```python
from build123d import *

# Parameters (mm, degrees)
SKETCH_1_R          = 3.15
EXTRUDE_1_DEPTH     = 2.15
SKETCH_2_R          = 2
EXTRUDE_2_DEPTH     = 35
CUT_EXTRUDE_1_DEPTH = 1.5


with BuildPart() as part:
    # 草图1 → 凸台-拉伸1 (new body)
    with BuildSketch(Plane(origin=(0, 0, 0), x_dir=(1, 0, 0), z_dir=(0, 1, 0))):
        Circle(SKETCH_1_R)
    extrude(amount=EXTRUDE_1_DEPTH)

    # 草图2 → 凸台-拉伸2 (add)
    with BuildSketch(Plane(origin=(0, 2.15, 0), x_dir=(1, 0, 0), z_dir=(0, 1, 0))):
        Circle(SKETCH_2_R)
    extrude(amount=EXTRUDE_2_DEPTH)

    # 草图3 → 切除-拉伸1 (cut)
    with BuildSketch(Plane.XZ):
        with BuildLine():
            Line((-0.5, 1), (-0.5, 2))
            Line((-0.5, 2), (0.5, 2))
            Line((0.5, 2), (0.5, 1))
            ThreePointArc((0.5, 1), (0.646446609, 0.646446609), (1, 0.5))
            Line((1, 0.5), (2, 0.5))
            Line((2, 0.5), (2, -0.5))
            Line((2, -0.5), (1, -0.5))
            ThreePointArc((1, -0.5), (0.646446609, -0.646446609), (0.5, -1))
            Line((0.5, -1), (0.5, -2))
            Line((0.5, -2), (-0.5, -2))
            Line((-0.5, -2), (-0.5, -1))
            ThreePointArc((-0.5, -1), (-0.646446609, -0.646446609), (-1, -0.5))
            Line((-1, -0.5), (-2, -0.5))
            Line((-2, -0.5), (-2, 0.5))
            Line((-2, 0.5), (-1, 0.5))
            ThreePointArc((-1, 0.5), (-0.646446609, 0.646446609), (-0.5, 1))
        make_face()
    extrude(amount=-CUT_EXTRUDE_1_DEPTH, mode=Mode.SUBTRACT)


solid = part.part
```
Here's how the part is built. I have some questions about the finished solid (model axes, mm). A direction names the side the tool comes from. Round coordinates to 2 decimals unless told otherwise and drop trailing zeros. Order: outer loops, then holes, each group sorted by start corner. A loop starts at its lowest first (then second) coordinate and runs counter-clockwise, first axis right, second up. Notation, with made-up numbers: M 4.5,42.5 L 15.5,42.5 A27 ccw 15.5,71.5 Z; hole C 16.25,88 d3. An arc over 180 degrees is marked long. Answer in a Markdown table with one row per item.
Item 1: Imagine slicing it at A-A, the plane x = 0. Write out the boundary of the cut face in (y, z), and give its area (3 significant figures).
A:
| item | result |
|---|---|
| outline | M 0,-3.15 L 2.15,-3.15 L 2.15,-2 L 37.15,-2 L 37.15,2 L 2.15,2 L 2.15,3.15 L 0,3.15 L 0,2 L 1.5,2 L 1.5,-2 L 0,-2 Z |
| area | 148 mm2 |
Item 2: Thinking about a two-plate mould opening in X: for faces 4 (the face through (1.5, 0.7, -0.5)), 5 (the face through (0, 19, 2)), 6 (the face through (-1.5, 0.7, 0.5)), 7 (the face through (1, 0, 1)), which applies, +X half, -X half, draft (parallel to the pull), parting line (faces both ways), or undercut?
A:
| item | result |
|---|---|
| face 4 | undercut |
| face 5 | parting line |
| face 6 | undercut |
| face 7 | draft |
Item 3: Imagine slicing it at B-B, the plane z = 0. Write out the boundary of the cut face in (x, y), and give its area (3 significant figures).
A:
| item | result |
|---|---|
| outline | M -3.15,0 L -2,0 L -2,1.5 L 2,1.5 L 2,0 L 3.15,0 L 3.15,2.15 L 2,2.15 L 2,37.15 L -2,37.15 L -2,2.15 L -3.15,2.15 Z |
| area | 148 mm2 |
Item 4: I'm going to push flat-ended pins straight in: pin 1 (1 mm diameter, centred on x = 1, y = 9.5, fed in from -Z); pin 2 (0.8 mm diameter, centred on y = 1, z = -1.5, fed in from -X); pin 3 (0.8 mm diameter, centred on x = 1.5, y = 0.5, fed in from +Z). Where does each tip first touch, or does it pass through?
A:
| item | result |
|---|---|
| pin 1 | stops at z = -1.94 |
| pin 2 | stops at x = -2.95 |
| pin 3 | stops at z = 2.95 |
Item 5: For faces 1 (the face through (-2.5, 1.06, 1.917)), 2 (the face through (0.5, 0.7, 1.5)), 3 (the face through (2, 2.15, 1)), which set-ups out of +Z, -Z, +X, -X, +Y, -Y let a thin tool reach every point of the face, with its end or its side?
A:
| item | result |
|---|---|
| face 1 | +Y, -Y |
| face 2 | -Y |
| face 3 | +Y |
Item 6: If I drill on L1, parallel to Y at x = -0.25, z = -2.5; L2, parallel to Y at x = -1.75, z = 0.25; L3, parallel to X at y = 28, z = -1, over which ranges is the centre line in solid material (lowest first)? Write a range as from..to.
A:
| item | result |
|---|---|
| L1 | y = 0..2.15 |
| L2 | y = 1.5..37.15 |
| L3 | x = -1.73..1.73 |
Item 7: Imagine slicing it at C-C, the plane y = 4. Write out the boundary of the cut face in (x, z).
A:
| item | result |
|---|---|
| outline | C 0,0 d4 |
